Here's how the part is built. I have some questions about the finished solid (model axes, mm). Face numbers are marked on the shaded views. A direction names the side the tool comes from. Round coordinates to 2 decimals unless told otherwise and drop trailing zeros. Loops run counter-clockwise (first coordinate to the right, second up) from the corner with the lowest first, then second, coordinate; pieces in that order, holes last. Notation, with made-up numbers: M 52.5,20 L 81.5,20 A32 ccw 81.5,52 Z; hole C 0,30 d9. An arc over 180 degrees is marked long. Use a Markdown table: item, result.
from build123d import *

# Parameters (mm, degrees)
EXTRUSION1_DEPTH        = 90
COQUE1_T                = -2.5
ESQUISSE2_R             = 10
ENL_V_MAT_EXTRU_1_DEPTH = 90
ESQUISSE3_R             = 10
ENL_V_MAT_EXTRU_2_DEPTH = 114.296072306


with BuildPart() as part:
    # Esquisse1 → Extrusion1 (new body)
    with BuildSketch(Plane.XY):
        with BuildLine():
            Line((40, -56), (-40, -56))
            Line((-40, -56), (-40, -19))
            Line((-40, -19), (-19.223282024, 12.627962156))
            ThreePointArc((-19.223282024, 12.627962156), (0, 23), (19.223282024, 12.627962156))
            Line((19.223282024, 12.627962156), (40, -19))
            Line((40, -19), (40, -56))
        make_face()
    extrude(amount=EXTRUSION1_DEPTH)

    # Coque1
    coque1_openings = [part.faces().sort_by_distance(p)[0] for p in [
        (40, -37.5, 45),
        (-40, -37.5, 45),
        (-29.611641012, -3.186018922, 45),
        (0, 23, 45),
        (29.611641012, -3.186018922, 45),
    ]]
    offset(amount=COQUE1_T, openings=coque1_openings, kind=Kind.INTERSECTION)

    # Esquisse2 → Enlèv. mat.-Extru.1 (cut)
    with BuildSketch(Plane.XZ.offset(56)):
        with Locations(Location((0, 45, 0), (0, 0, 270))):
            Circle(ESQUISSE2_R)
    extrude(amount=-ENL_V_MAT_EXTRU_1_DEPTH, mode=Mode.SUBTRACT)

    # Esquisse3 → Enlèv. mat.-Extru.2 (cut, through all)
    with BuildSketch(Plane(origin=(0, 0, 0), x_dir=(-1, 0, 0), z_dir=(0, 0, -1))):
        Circle(ESQUISSE3_R)
    extrude(amount=-ENL_V_MAT_EXTRU_2_DEPTH, mode=Mode.SUBTRACT)


solid = part.part
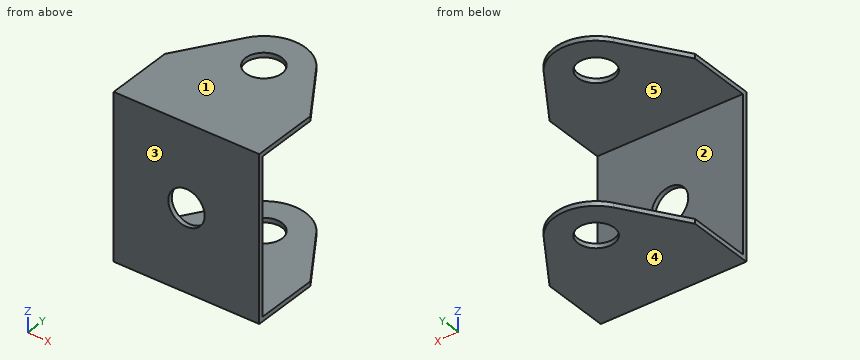
1. We'd pull the mould along Z, two halves only. Please class the marked faces 3, 4 and 5: +Z half, -Z half, draft (parallel to the pull), parting line (faces both ways), or undercut.
Answer sheet:
| item | result |
|---|---|
| face 3 | draft |
| face 4 | -Z half |
| face 5 | undercut |
2. I need wall thicknesses on probe 1 along X at (y, z) = (-54.15, 45); probe 2 along Z at (x, y) = (-29.5, -11.5); probe 3 along Y at (x, z) = (0, 88). Which ranges of each line are inside material? Lowest first, please. Write a range as from..to.
Answer sheet:
| item | result |
|---|---|
| probe 1 | -40..-10, 10..40 |
| probe 2 | 0..2.5, 87.5..90 |
| probe 3 | -56..-10, 10..23 |
3. Which directions (+Z, -Z, +X, -X, +Y, -Y) give clear straight access to the entire face, cutting with the end or side of a thin tool? Please do the marked faces 1 and 2.
Answer sheet:
| item | result |
|---|---|
| face 1 | +Z, +X, -X, +Y, -Y |
| face 2 | +X, -X, +Y |
4. Imagine slicing it at A-A, the plane y = -28. Write out the boundary of the cut face in (x, z), then the cut area to 3 significant figures.
Answer sheet:
| item | result |
|---|---|
| outline | M -40,0 L 40,0 L 40,2.5 L -40,2.5 Z; M -40,87.5 L 40,87.5 L 40,90 L -40,90 Z |
| area | 400 mm2 |
5. Imagine slicing it at B-B, the plane x = 0. Write out the boundary of the cut face in (y, z), then the cut area to 4 significant figures.
Answer sheet:
| item | result |
|---|---|
| outline | M -56,0 L -10,0 L -10,2.5 L -53.5,2.5 L -53.5,35 L -56,35 Z; M -56,55 L -53.5,55 L -53.5,87.5 L -10,87.5 L -10,90 L -56,90 Z; M 10,0 L 23,0 L 23,2.5 L 10,2.5 Z; M 10,87.5 L 23,87.5 L 23,90 L 10,90 Z |
| area | 457.5 mm2 |
6. Imagine slicing it at C-C, the plane z = 45. Write out the boundary of the cut face in (x, y), then the cut area to 3 significant figures.
Answer sheet:
| item | result |
|---|---|
| outline | M -40,-56 L -10,-56 L -10,-53.5 L -40,-53.5 Z; M 10,-56 L 40,-56 L 40,-53.5 L 10,-53.5 Z |
| area | 150 mm2 |
7. For pin 1 Ø12 at (x, z) = (2.5, 20.5) entering from +Y, with a flat end and sliding along its axis, tell me the tip position at first contact or that it passes through.
Answer sheet:
| item | result |
|---|---|
| pin 1 | y = -53.5 |
8. Imagine slicing it at D-D, the plane y = 0. Write out the boundary of the cut face in (x, z).
Answer sheet:
| item | result |
|---|---|
| outline | M -27.52,0 L -10,0 L -10,2.5 L -27.52,2.5 Z; M -27.52,87.5 L -10,87.5 L -10,90 L -27.52,90 Z; M 10,0 L 27.52,0 L 27.52,2.5 L 10,2.5 Z; M 10,87.5 L 27.52,87.5 L 27.52,90 L 10,90 Z |
